Check sheet for the modelled part. Datum: model origin and axes. Units: mm. Face numbers are marked on the shaded views. A direction names the side the tool comes from. Give positions to 0.01 mm unless a question says otherwise; leave off trailing zeros. Order: outer loops, then holes, each group sorted by start corner. A loop starts at its lowest first (then second) coordinate and runs counter-clockwise, first axis right, second up.
Item 1: Access from +Z, -Z, +X, -X, +Y, -Y to the whole of each face (thin tool, end or side, straight path). Record for the marked faces 1, 2 and 3.
Item 2: Release check for a two-part mould opening along Z. For the marked faces 4, 5, 6 and 7 record: released by +Z, released by -Z, zero draft, split by the parting line, or undercut.
Item 3: Gauge pin test, flat ends, axial feed: P1, Ø2, axis at y = 2, z = 11.5, coming from the -X side; P2, Ø0.6, axis at x = 7, z = 13.5, coming from the +Y side; P3, Ø1.6, axis at x = -7.5, z = 12.5, coming from the -Y side; P4, Ø7, axis at x = 0, y = 0, coming from the -Z side. Record the tip position at first contact, or that the pin passes through.
Item 4: Material ranges on line 1 along Z through (x, y) = (6.5, 2.5); line 2 along Z through (x, y) = (-0.5, -6.5); line 3 along X through (y, z) = (0, -4.75), recorded low to high.
Item 5: Sectioned sample at D-D on y = 3. Count the separate pieces of the cut face and the enclosed holes in it, and give its area (3 significant figures).
Item 6: Sectioned sample at C-C on z = 6. Record the boundary of the cut face in (x, y).
Item 7: Sectioned sample at A-A on x = 0. Record the boundary of the cut face in (y, z).
Item 8: Sectioned sample at B-B on y = 0. Record the boundary of the cut face in (x, z), and give its area (3 significant figures).
from build123d import *

# Parameters (mm, degrees)
F3_DEPTH = 25
F4_DEPTH = 25


with BuildPart() as f1:
    # F0 (on Right) → F1 (revolve)
    with BuildSketch(Plane.YZ):
        Polygon((6.75, 16), (6.75, 4), (6.75, 3.3), (4.5, 3.3), (4.5, 0), (4.5, -19.3), (6, -18.6), (7.5, -15.6), (6, -15.6), (7.6, -12.6), (6, -12.6), (7.7, -8.6), (6, -8.6), (6, -2.6), (8.75, 0), (8.75, 16), align=None)
    revolve(axis=Axis((0, 0, 14.120129), (0, 0, 1)))

    # F2 (on Right) → F3 (cut)
    with BuildSketch(Plane.YZ):
        Polygon((-1.55, 11.05), (-1.55, 8), (1.55, 8.014865), (1.55, 11.05), (1.55, 16.095196), (-1.55, 16.095196), align=None)
        Polygon((-2.367748, 8), (-1.55, 8), (-1.55, 11.05), (-5.562683, 11.333183), (-5.562683, 11.072353), (-5.579271, 8.226643), align=None)
    extrude(amount=F3_DEPTH, mode=Mode.SUBTRACT)

    # F2 (on Right) → F4 (cut)
    with BuildSketch(Plane.YZ):
        Polygon((1.55, 11.05), (1.55, 8.014865), (1.55, 8), (2.367748, 8), (5.579271, 8.226643), (5.562683, 11.072353), (5.562683, 11.333183), align=None)
        Polygon((-1.55, 11.05), (-1.55, 8), (1.55, 8.014865), (1.55, 11.05), (1.55, 16.095196), (-1.55, 16.095196), align=None)
    extrude(amount=-F4_DEPTH, mode=Mode.SUBTRACT)


solid = f1.part
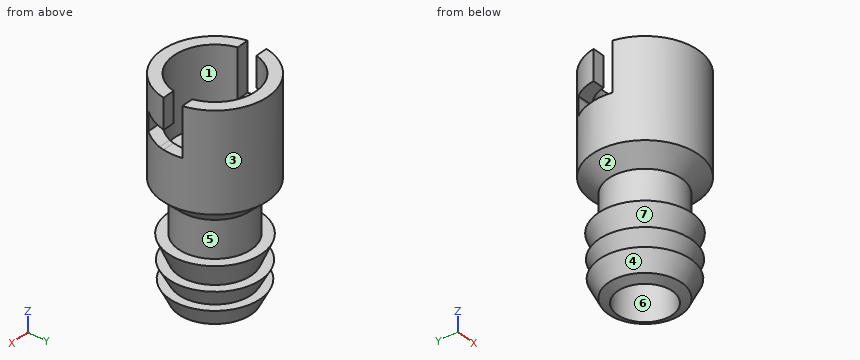
Report:
1. face 1: +Z
1. face 2: none
1. face 3: +Z, -Z
2. face 4: released by -Z
2. face 5: undercut
2. face 6: zero draft
2. face 7: undercut
3. P1: stops at x = -8.61
3. P2: stops at y = 5.63
3. P3: stops at y = -5.63
3. P4: passes through
4. line 1: z = -16.67 to -15.6, -13.79 to -12.6, -10.33 to -8.6, -1.69 to 16
4. line 2: z = -17.56 to -15.6, -14.63 to -12.6, -11.38 to -8.6, -2.11 to 3.3
4. line 3: x = -6 to -4.5, 4.5 to 6
5. separate pieces: 3
5. enclosed holes: 0
5. area: 177 mm2
6. outline: circle Ø17.5 at (0, 0); hole circle Ø13.5 at (0, 0)
7. outline: (-8.75, 0) - (-6, -2.6) - (-6, -8.6) - (-7.7, -8.6) - (-6, -12.6) - (-7.6, -12.6) - (-6, -15.6) - (-7.5, -15.6) - (-6, -18.6) - (-4.5, -19.3) - (-4.5, 3.3) - (-6.75, 3.3) - (-6.75, 16) - (-8.75, 16) - close; (4.5, -19.3) - (6, -18.6) - (7.5, -15.6) - (6, -15.6) - (7.6, -12.6) - (6, -12.6) - (7.7, -8.6) - (6, -8.6) - (6, -2.6) - (8.75, 0) - (8.75, 16) - (6.75, 16) - (6.75, 3.3) - (4.5, 3.3) - close
8. outline: (-8.75, 0) - (-6, -2.6) - (-6, -8.6) - (-7.7, -8.6) - (-6, -12.6) - (-7.6, -12.6) - (-6, -15.6) - (-7.5, -15.6) - (-6, -18.6) - (-4.5, -19.3) - (-4.5, 3.3) - (-6.75, 3.3) - (-6.75, 8.01) - (-8.75, 8.01) - close; (4.5, -19.3) - (6, -18.6) - (7.5, -15.6) - (6, -15.6) - (7.6, -12.6) - (6, -12.6) - (7.7, -8.6) - (6, -8.6) - (6, -2.6) - (8.75, 0) - (8.75, 8.01) - (6.75, 8.01) - (6.75, 3.3) - (4.5, 3.3) - close
8. area: 127 mm2
